Can you work these out from the model? Positions are in its coordinate system, mm. Face numbers are marked on the shaded views. A direction names the side the tool comes from. Coordinates: 2 decimals unless noted, no trailing zeros. Write each loop counter-clockwise with the first axis right and the second up, starting at its lowest first coordinate (ties: lowest second). Pieces come first, ordered by that corner, then holes. Notation, with made-up numbers: (46, 43.25) - (93, 43.25) arc R16 cw to (93, 47.25) - close; hole circle Ø6 at (41.25, 65). An arc over 180 degrees is marked (long way). Use one line per item in the form item = value. Start each with the question number.
(1) If we section it at A-A on x = 190.7: Please give me the cut outline in (y, z).
(2) If we section it at C-C on z = 6: Please give me the cut outline in (x, y).
(3) If I drill on probe 1 along Y at (x, z) = (190, 3); probe 2 along X at (y, z) = (-11, 3); probe 3 along X at (y, z) = (-11, 6), over which ranges is the centre line in solid material (lowest first)? Write a range as from..to.
(4) For pin 1 Ø11 at (x, z) = (39, 3) entering from -Y; pin 2 Ø5 at (y, z) = (-42.5, -4) entering from -X; pin 3 Ø17 at (x, y) = (70, -11.1) entering from -Z, each with a flat end and sliding along its axis, tell me the tip position at first contact or that it passes through.
(5) If we section it at D-D on x = 87: Please give me the cut outline in (y, z).
(6) On a 3-axis mill with a long thin cutter (end or side, diameter ignored), from which of +Z, -Z, +X, -X, +Y, -Y can I reach the whole of each face in a straight line? I mean the marked faces 1 and 2. Say none if no direction works.
(7) If we section it at B-B on y = -49: Please give me the cut outline in (x, z).
```python
from build123d import *

# Parameters (mm, degrees)
PAD_DEPTH    = 10
PAD001_DEPTH = 60
SKETCH003_W  = 10
SKETCH003_H  = 10
PAD003_DEPTH = 60
PAD004_DEPTH = 10
SKETCH005_R  = 6.5
HOLE_DEPTH   = 34.201


with BuildPart() as part:
    # Sketch → Pad (new body)
    with BuildSketch(Plane.XZ):
        Polygon((0, 0), (223, 0), (227.6, -24.2), (237.424096, -22.33261), (231.278228, 10), (0, 10), align=None)
    extrude(amount=PAD_DEPTH)

    # Sketch001 → Pad001 (join)
    with BuildSketch(Plane.XZ.offset(10)):
        Polygon((223, 0), (227.6, -24.2), (237.424096, -22.33261), (231.278228, 10), (223, 10), align=None)
    extrude(amount=PAD001_DEPTH)

    # Sketch003 → Pad003 (join)
    with BuildSketch(Plane.XZ.offset(10)):
        with Locations((5, 5)):
            Rectangle(SKETCH003_W, SKETCH003_H)
    extrude(amount=PAD003_DEPTH)

    # Sketch004 → Pad004 (join)
    with BuildSketch(Plane.XY):
        with BuildLine():
            ThreePointArc((58.69456, -17.832638), (70, -25), (81.30544, -17.832638))
            Line((85, -10), (81.30544, -17.832638))
            Line((85, 0), (85, -10))
            Line((55, 0), (85, 0))
            Line((55, -10), (55, 0))
            Line((55, -10), (58.69456, -17.832638))
        make_face()
        with BuildLine():
            Line((179.39456, -17.832638), (175.7, -10))
            Line((175.7, -10), (175.7, 0))
            Line((175.7, 0), (205.7, 0))
            Line((205.7, 0), (205.7, -10))
            Line((205.7, -10), (202.00544, -17.832638))
            ThreePointArc((179.39456, -17.832638), (190.7, -25), (202.00544, -17.832638))
        make_face()
    extrude(amount=PAD004_DEPTH)

    # Sketch005 → Hole (cut, through all)
    with BuildSketch(Plane.XY.offset(10)):
        with Locations((70, -11.1)):
            Circle(SKETCH005_R)
        with Locations((190.7, -11.1)):
            Circle(SKETCH005_R)
    extrude(amount=-HOLE_DEPTH, mode=Mode.SUBTRACT)


solid = part.part
```
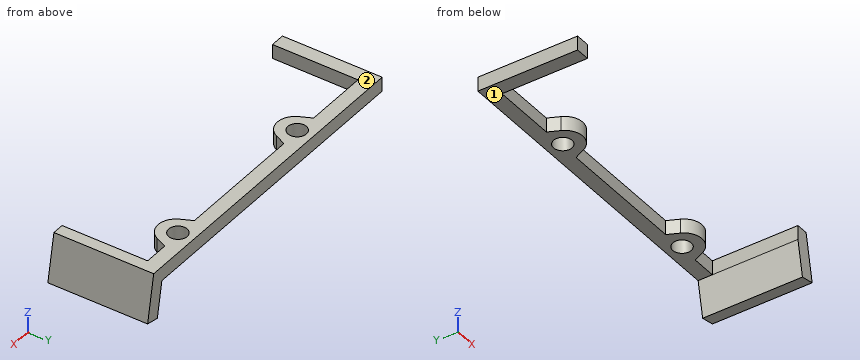
Reported:
q1.outline = (-25, 0) - (-17.6, 0) - (-17.6, 10) - (-25, 10) - close; (-4.6, 0) - (0, 0) - (0, 10) - (-4.6, 10) - close
q2.outline = (0, -70) - (10, -70) - (10, -10) - (55, -10) - (58.69, -17.83) arc R12.5 ccw to (81.31, -17.83) - (85, -10) - (175.7, -10) - (179.39, -17.83) arc R12.5 ccw to (202.01, -17.83) - (205.7, -10) - (223, -10) - (223, -70) - (232.04, -70) - (232.04, 0) - (0, 0) - close; hole circle Ø13 at (70, -11.1); hole circle Ø13 at (190.7, -11.1)
q3.probe_1 = -24.98..-17.56, -4.64..0
q3.probe_2 = 0..10, 55.47..63.5, 76.5..84.53, 176.17..184.2, 197.2..205.23, 223..232.61
q3.probe_3 = 0..10, 55.47..63.5, 76.5..84.53, 176.17..184.2, 197.2..205.23, 223..232.04
q4.pin_1 = -10
q4.pin_2 = 223.29
q4.pin_3 = 0
q5.outline = (-10, 0) - (0, 0) - (0, 10) - (-10, 10) - close
q6.face_1 = -Z, -X, +Y, -Y
q6.face_2 = +Z, +X, -X, +Y, -Y
q7.outline = (0, 0) - (10, 0) - (10, 10) - (0, 10) - close; (223, 0) - (227.6, -24.2) - (237.42, -22.33) - (231.28, 10) - (223, 10) - close
